from build123d import *

# Parameters (mm, degrees)
BOSS_EXTRUDE1_DEPTH = 0.35
FILLET1_R           = 10


with BuildPart() as part:
    # Sketch1 → Boss-Extrude1 (new body)
    with BuildSketch(Plane(origin=(0, 0, 0.002129552), x_dir=(1, 0, 0), z_dir=(0, 1, 0))):
        Polygon((65.957189, 129.495721477), (66.457189, 132.495721477), (66.457189, 139.495721477), (65.957189, 142.495721477), (65.957189, 143.495721477), (64.457189, 143.495721477), (64.457189, 142.495721477), (63.957189, 139.495721477), (63.957189, 132.495721477), (64.457189, 129.495721477), (64.457189, 128.495721477), (65.207189, 128.495721477), (65.957189, 128.495721477), align=None)
    extrude(amount=BOSS_EXTRUDE1_DEPTH)

    # Fillet1
    fillet1_edges = [part.edges().sort_by_distance(p)[0] for p in [
        (66.457189, 0.175, -132.493591924),
        (63.957189, 0.175, -132.493591924),
        (63.957189, 0.175, -139.493591924),
        (66.457189, 0.175, -139.493591924),
    ]]
    fillet(fillet1_edges, radius=FILLET1_R)


solid = part.part
Source: CAD feature listing. Evaluate the final solid. Frame: model axes, mm. Round coordinates to 2 decimals unless told otherwise and drop trailing zeros. Loops run counter-clockwise (first coordinate to the right, second up) from the corner with the lowest first, then second, coordinate; pieces in that order, holes last. Notation, with made-up numbers: (47.5, -10.75) - (75.5, -10.75) arc R11 cw to (75.5, 3.25) - close; hole circle Ø3 at (73, 35). An arc over 180 degrees is marked (long way). Write item = value, one per line. Start each with the question number.
(1) Section query C-C, the plane z = -141.25. Output: boundary loops of the cut face in (x, y).
(2) Ray query, line 1 along X through (y, z) = (0.1, -142.5); line 2 along X through (y, z) = (0.3, -141.5). Return the intervals inside material, ascending. Write a range as from..to.
(3) Section query A-A, the plane y = 0.2. Output: boundary loops of the cut face in (x, z), plus the area to 3 significant figures.
(4) Section query B-B, the plane z = -132.5. Output: boundary loops of the cut face in (x, y), plus the area to 3 significant figures.
Conclusion:
q1.outline = (64.25, 0) - (66.16, 0) - (66.16, 0.35) - (64.25, 0.35) - close
q2.line_1 = 64.46..65.96
q2.line_2 = 64.29..66.12
q3.outline = (63.96, -138.67) arc R10 ccw to (64.09, -140.31) - (64.46, -142.49) - (64.46, -143.49) - (65.96, -143.49) - (65.96, -142.49) - (66.32, -140.31) arc R10 ccw to (66.46, -138.67) - (66.46, -133.32) arc R10 ccw to (66.32, -131.68) - (65.96, -129.49) - (65.96, -128.49) - (64.46, -128.49) - (64.46, -129.49) - (64.09, -131.68) arc R10 ccw to (63.96, -133.32) - close
q3.area = 32.4 mm2
q4.outline = (63.99, 0) - (66.42, 0) - (66.42, 0.35) - (63.99, 0.35) - close
q4.area = 0.851 mm2
